Print and shaded views of the part. All mm, measured from the part's lowest x, y and z. A direction names the side the tool comes from. Coordinates: 2 decimals unless noted, no trailing zeros. Order: outer loops, then holes, each group sorted by start corner. A loop starts at its lowest first (then second) coordinate and runs counter-clockwise, first axis right, second up. Notation, with made-up numbers: (69.25, 64) -> (97.25, 64) arc R9 ccw to (97.25, 70) -> close; hole circle Ø5 at (89, 81). An arc over 180 degrees is marked (long way). Return JSON: item names as keys, results as strings. Group by question number.
1) Cut at D-D (x = 86). Write the cut outline in (y, z), and give its area (3 significant figures).
2) Cut at C-C (z = 141). Write the cut outline in (x, y), and give its area (3 significant figures).
3) Which spindle directions (+Z, -Z, +X, -X, +Y, -Y) get a long thin tool onto all of the face, cutting with end or side? Do the marked faces 4, 5 and 6. Say none if no direction does.
4) Probe line 1 (X direction, y = 17.25, z = 45); line 2 (X direction, y = 11.25, z = 24); line 3 (X direction, y = 20.25, z = 85.5). List the from-to ranges inside material, lowest first.
5) Flat gauge pin, fed straight in: pin 1 (1 mm diameter, centred on x = 40, z = 130.5, fed in from -Y). Where does the tip first touch, or does it go through?
6) Cut at A-A (y = 16.25). Write the cut outline in (x, z).
7) Cut at B-B (y = 5). Write the cut outline in (x, z).
8) Pull direction X, two halves, no side cores. Call the marked faces 1, 2 and 3: +X half, -X half, draft (parallel to the pull), parting line (faces both ways), or undercut.
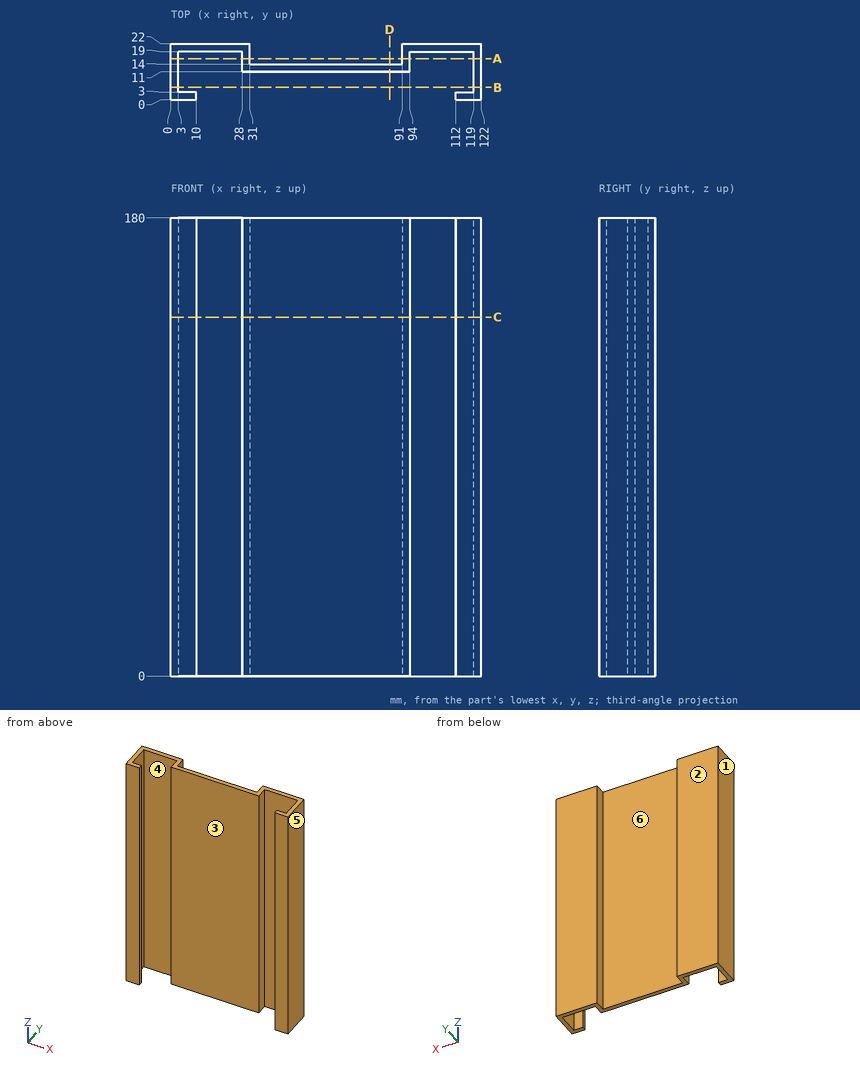
Answers below:
{
 "1": {"outline": "(11, 0) -> (14, 0) -> (14, 180) -> (11, 180) -> close", "area": "540 mm^2"},
 "2": {"outline": "(0, 0) -> (10, 0) -> (10, 3) -> (3, 3) -> (3, 19) -> (28, 19) -> (28, 11) -> (94, 11) -> (94, 19) -> (119, 19) -> (119, 3) -> (112, 3) -> (112, 0) -> (122, 0) -> (122, 22) -> (91, 22) -> (91, 14) -> (31, 14) -> (31, 22) -> (0, 22) -> close", "area": "570 mm^2"},
 "3": {"face 4": "+Z, -Z", "face 5": "+Z, -Z, +X, +Y, -Y", "face 6": "+Z, -Z, +Y"},
 "4": {"line 1": "x = 0 to 3, 28 to 31, 91 to 94, 119 to 122", "line 2": "x = 0 to 3, 28 to 94, 119 to 122", "line 3": "x = 0 to 31, 91 to 122"},
 "5": {"pin 1": "stops at y = 11"},
 "6": {"outline": "(0, 0) -> (3, 0) -> (3, 180) -> (0, 180) -> close; (28, 0) -> (31, 0) -> (31, 180) -> (28, 180) -> close; (91, 0) -> (94, 0) -> (94, 180) -> (91, 180) -> close; (119, 0) -> (122, 0) -> (122, 180) -> (119, 180) -> close"},
 "7": {"outline": "(0, 0) -> (3, 0) -> (3, 180) -> (0, 180) -> close; (119, 0) -> (122, 0) -> (122, 180) -> (119, 180) -> close"},
 "8": {"face 1": "-X half", "face 2": "draft", "face 3": "undercut"}
}
